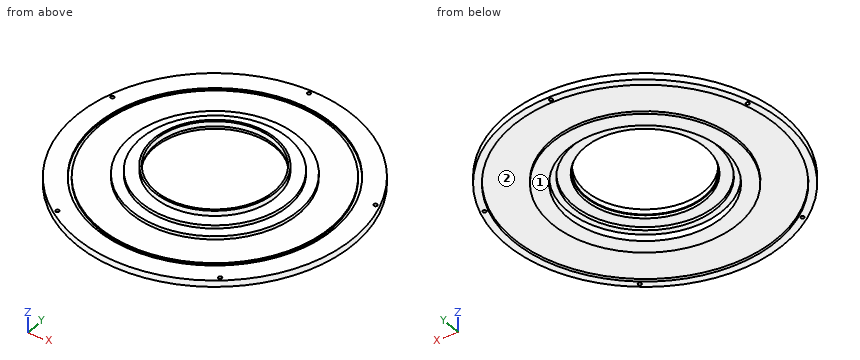
```python
from build123d import *

# Parameters (mm, degrees)
SKETCH1_R         = 215
SKETCH1_R_2       = 120
PLATE_DEPTH       = 10
SKETCH2_R         = 130
SKETCH2_R_2       = 111
BELLMOUTH1_DEPTH  = 5
SKETCH3_R         = 114
SKETCH3_R_2       = 93
BELLMOUTH2_DEPTH  = 5
SKETCH4_R         = 94.5
SKETCH4_R_2       = 91.5
BELLMOUTH3_DEPTH  = 8
SKETCH5_R         = 204
SKETCH5_R_2       = 144
COMB_GROOVE_DEPTH = 4
SKETCH6_R         = 184
SKETCH6_R_2       = 179
BAND_SEAT_DEPTH   = 3
SKETCH7_R         = 2.75
ROD_HOLES_DEPTH   = 10


with BuildPart() as part:
    # Sketch1 → Plate (new body)
    with BuildSketch(Plane.XY):
        Circle(SKETCH1_R)
        Circle(SKETCH1_R_2, mode=Mode.SUBTRACT)
    extrude(amount=PLATE_DEPTH)

    # Sketch2 → Bellmouth1 (add)
    with BuildSketch(Plane.XY.offset(10)):
        Circle(SKETCH2_R)
        Circle(SKETCH2_R_2, mode=Mode.SUBTRACT)
    extrude(amount=BELLMOUTH1_DEPTH)

    # Sketch3 → Bellmouth2 (add)
    with BuildSketch(Plane.XY.offset(15)):
        Circle(SKETCH3_R)
        Circle(SKETCH3_R_2, mode=Mode.SUBTRACT)
    extrude(amount=BELLMOUTH2_DEPTH)

    # Sketch4 → Bellmouth3 (add)
    with BuildSketch(Plane.XY.offset(20)):
        Circle(SKETCH4_R)
        Circle(SKETCH4_R_2, mode=Mode.SUBTRACT)
    extrude(amount=BELLMOUTH3_DEPTH)

    # Sketch5 → Comb_groove (cut)
    with BuildSketch(Plane.XY):
        Circle(SKETCH5_R)
        Circle(SKETCH5_R_2, mode=Mode.SUBTRACT)
    extrude(amount=COMB_GROOVE_DEPTH, mode=Mode.SUBTRACT)

    # Sketch6 → Band_seat (cut)
    with BuildSketch(Plane.XY.offset(7)):
        Circle(SKETCH6_R)
        Circle(SKETCH6_R_2, mode=Mode.SUBTRACT)
    extrude(amount=BAND_SEAT_DEPTH, mode=Mode.SUBTRACT)

    # Sketch7 → Rod_holes (cut)
    with BuildSketch(Plane.XY):
        with Locations((198.770811906, 64.584551824)):
            Circle(SKETCH7_R)
        with Locations((0, 209)):
            Circle(SKETCH7_R)
        with Locations((-198.770811906, 64.584551824)):
            Circle(SKETCH7_R)
        with Locations((-122.847117729, -169.084551824)):
            Circle(SKETCH7_R)
        with Locations((122.847117729, -169.084551824)):
            Circle(SKETCH7_R)
    extrude(amount=ROD_HOLES_DEPTH, mode=Mode.SUBTRACT)


solid = part.part
```
The model under review builds one solid part; all positions refer to its coordinate system, in mm. Face numbers are marked on the shaded views. Round coordinates to 2 decimals unless told otherwise and drop trailing zeros. Put each result on its own line as item: value.
Q1. To check wall thickness, follow L1, parallel to Y at x = 0, z = 6.25; L2, parallel to Y at x = 0, z = 1.95; L3, parallel to X at y = -120.5, z = 2. State the ranges of each line that lie inside material, in increasing order.
Result set:
L1: y = -215 to -120, 120 to 206.25, 211.75 to 215
L2: y = -215 to -204, -144 to -120, 120 to 144, 204 to 206.25, 211.75 to 215
L3: x = -178.06 to -164.61, -78.84 to 78.84, 164.61 to 178.06
Q2. For pin 1 (4 mm diameter, centred on y = 25, z = 13, fed in from +X); pin 2 (8 mm diameter, centred on x = -17, z = 15.5, fed in from -Y); pin 3 (10 mm diameter, centred on x = 41.5, z = 13.5, fed in from +Y); pin 4 (4.5 mm diameter, centred on x = 0, y = 209, fed in from +Z), all flat-tipped, find the tip position at first contact; note any pin that passes through.
Result set:
pin 1: stops at x = 127.95
pin 2: stops at y = -129.35
pin 3: stops at y = 211.63
pin 4: passes through
Q3. Mouldability with a two-part tool opening along Y and no side actions: class the marked faces 1 and 2 as released by +Y, released by -Y, zero draft, split by the parting line, or undercut.
Result set:
face 1: zero draft
face 2: undercut
